Can you work these out from the model? Positions are in its coordinate system, mm. A direction names the side the tool comes from. Give positions to 0.01 mm unless a question says otherwise; leave off trailing zeros. Order: outer loops, then holes, each group sorted by start corner. A loop starts at its lowest first (then second) coordinate and runs counter-clockwise, first axis right, second up. Notation, with made-up numbers: (70.25, 70.25) - (120.25, 70.25) arc R30 cw to (120.25, 105.25) - close; hole circle Ø8 at (40.25, 47). An arc over 180 degrees is marked (long way). Return JSON: item names as keys, results as strings.
```python
from build123d import *

# Parameters (mm, degrees)
RESSALTO_EXTRUS_O1_DEPTH = 5
ESBO_O2_R                = 2.5
CORTE_EXTRUS_O1_DEPTH    = 5
CORTE_EXTRUS_O2_DEPTH    = 10


with BuildPart() as part:
    # Esboço1 → Ressalto-extrusão1 (new body)
    with BuildSketch(Plane(origin=(0, 0, 0), x_dir=(1, 0, 0), z_dir=(0, 1, 0))):
        with BuildLine():
            Line((68.172006189, -100), (-18.172006189, -100))
            ThreePointArc((-18.172006189, -100), (-32.132026705, -95.739282224), (-41.333670617, -84.409426174))
            Line((-41.333670617, -84.409426174), (-98.161664428, 55.474866284))
            ThreePointArc((-98.161664428, 55.474866284), (-99.536112271, 60.090630534), (-100, 64.884292458))
            Line((-100, 64.884292458), (-100, 90))
            ThreePointArc((-100, 90), (-97.071067812, 97.071067812), (-90, 100))
            Line((-90, 100), (140, 100))
            ThreePointArc((140, 100), (147.071067812, 97.071067812), (150, 90))
            Line((150, 90), (150, 64.884292458))
            ThreePointArc((150, 64.884292458), (149.536112271, 60.090630534), (148.161664428, 55.474866284))
            Line((148.161664428, 55.474866284), (91.333670617, -84.409426174))
            ThreePointArc((91.333670617, -84.409426174), (82.132026705, -95.739282224), (68.172006189, -100))
        make_face()
    extrude(amount=RESSALTO_EXTRUS_O1_DEPTH)

    # Esboço2 → Corte-extrusão1 (cut)
    with BuildSketch(Plane(origin=(0, 5, 0), x_dir=(1, 0, 0), z_dir=(0, 1, 0))):
        with Locations(Location((-85, 85, 0), (0, 0, 270))):
            Circle(ESBO_O2_R)
        with Locations(Location((-10, -85, 0), (0, 0, 270))):
            Circle(ESBO_O2_R)
        with Locations(Location((60, -85, 0), (0, 0, 270))):
            Circle(ESBO_O2_R)
        with Locations(Location((135, 85, 0), (0, 0, 270))):
            Circle(ESBO_O2_R)
    extrude(amount=-CORTE_EXTRUS_O1_DEPTH, mode=Mode.SUBTRACT)

    # Esboço3 → Corte-extrusão2 (cut)
    with BuildSketch(Plane(origin=(0, 5, 0), x_dir=(1, 0, 0), z_dir=(0, 1, 0))):
        with BuildLine():
            Line((-21.5212831, 26.23622953), (2.8537169, -33.76377047))
            ThreePointArc((2.8537169, -33.76377047), (6.534374465, -38.29571289), (12.118382671, -40))
            Line((12.118382671, -40), (37.881617329, -40))
            ThreePointArc((37.881617329, -40), (43.465625535, -38.29571289), (47.1462831, -33.76377047))
            Line((47.1462831, -33.76377047), (71.5212831, 26.23622953))
            ThreePointArc((71.5212831, 26.23622953), (70.552330218, 35.584008207), (62.256617329, 40))
            Line((62.256617329, 40), (-12.256617329, 40))
            ThreePointArc((-12.256617329, 40), (-20.552330218, 35.584008207), (-21.5212831, 26.23622953))
        make_face()
    extrude(amount=-CORTE_EXTRUS_O2_DEPTH, mode=Mode.SUBTRACT)


solid = part.part
```
1. Suppose I cut it at D-D (x = 107.5). List the corners of the cut face in (y, z) for me, plus the area to 3 significant figures.
Checks:
{"outline": "(0, -100) - (5, -100) - (5, 44.62) - (0, 44.62) - close", "area": "723 mm^2"}
2. Suppose I cut it at C-C (z = -18.5). List the corners of the cut face in (x, y) for me.
Checks:
{"outline": "(-83.14, 0) - (-18.38, 0) - (-18.38, 5) - (-83.14, 5) - close; (68.38, 0) - (133.14, 0) - (133.14, 5) - (68.38, 5) - close"}
3. If I drill on L1, parallel to X at y = 2.9, z = -83.5; L2, parallel to Z at x = 19, y = 2.05; L3, parallel to Z at x = 5.5, y = 2.25, over which ranges is the centre line in solid material (lowest first)? Write a range as [from, to].
Checks:
{"L1": "[-100, -87], [-83, 133], [137, 150]", "L2": "[-100, -40], [40, 100]", "L3": "[-100, -40], [37.5, 100]"}
4. For pin 1 Ø3 at (y, z) = (3, -0.5) entering from +X; pin 2 Ø2 at (y, z) = (3.5, -8.5) entering from -X; pin 3 Ø3 at (x, z) = (135, -85) entering from -Y, each with a flat end and sliding along its axis, tell me the tip position at first contact or that it passes through.
Checks:
{"pin 1": "x = 126.44", "pin 2": "x = -79.48", "pin 3": "through"}
5. Suppose I cut it at A-A (x = 32). List the corners of the cut face in (y, z) for me.
Checks:
{"outline": "(0, -100) - (5, -100) - (5, -40) - (0, -40) - close; (0, 40) - (5, 40) - (5, 100) - (0, 100) - close"}
6. Suppose I cut it at B-B (y = 2.4). List the corners of the cut face in (x, z) for me.
Checks:
{"outline": "(-100, -90) arc R10 ccw to (-90, -100) - (140, -100) arc R10 ccw to (150, -90) - (150, -64.88) arc R25 ccw to (148.16, -55.47) - (91.33, 84.41) arc R25 ccw to (68.17, 100) - (-18.17, 100) arc R25 ccw to (-41.33, 84.41) - (-98.16, -55.47) arc R25 ccw to (-100, -64.88) - close; hole circle Ø5 at (-85, -85); hole (-21.52, -26.24) arc R10 ccw to (-12.26, -40) - (62.26, -40) arc R10 ccw to (71.52, -26.24) - (47.15, 33.76) arc R10 ccw to (37.88, 40) - (12.12, 40) arc R10 ccw to (2.85, 33.76) - close; hole circle Ø5 at (-10, 85); hole circle Ø5 at (60, 85); hole circle Ø5 at (135, -85)"}
7. Thinking about a two-plate mould opening in X: for faces 1 (the face through (82.304, 2.465, 95.623)), 2 (the face through (137.48, 2.54, -85.33)), 3 (the face through (23, 2, -100)), 4 (the face through (-100, 2, -77)), which applies, +X half, -X half, draft (parallel to the pull), parting line (faces both ways), or undercut?
Checks:
{"face 1": "+X half", "face 2": "undercut", "face 3": "draft", "face 4": "-X half"}
8. On a 3-axis mill with a long thin cutter (end or side, diameter ignored), from which of +Z, -Z, +X, -X, +Y, -Y can I reach the whole of each face in a straight line? I mean faces 5 (the face through (-97.15, 2.46, -96.99)), 6 (the face through (26, 3, -40)). Say none if no direction works.
Checks:
{"face 5": "-Z, -X, +Y, -Y", "face 6": "+Y, -Y"}
